The figure shows three views and two pictorial views of one solid part (mm, origin at its lowest corner). Answer the questions. Give positions to 0.01 mm unless a question says otherwise; leave off trailing zeros. Order: outer loops, then holes, each group sorted by start corner. A loop starts at its lowest first (then second) coordinate and runs counter-clockwise, first axis right, second up. Notation, with made-up numbers: (35.5, -11) -> (51.5, -11) arc R19 ccw to (51.5, -6) -> close; hole circle Ø11 at (70.25, -33). An arc over 180 degrees is marked (long way). Use one line per item in the form item = value.
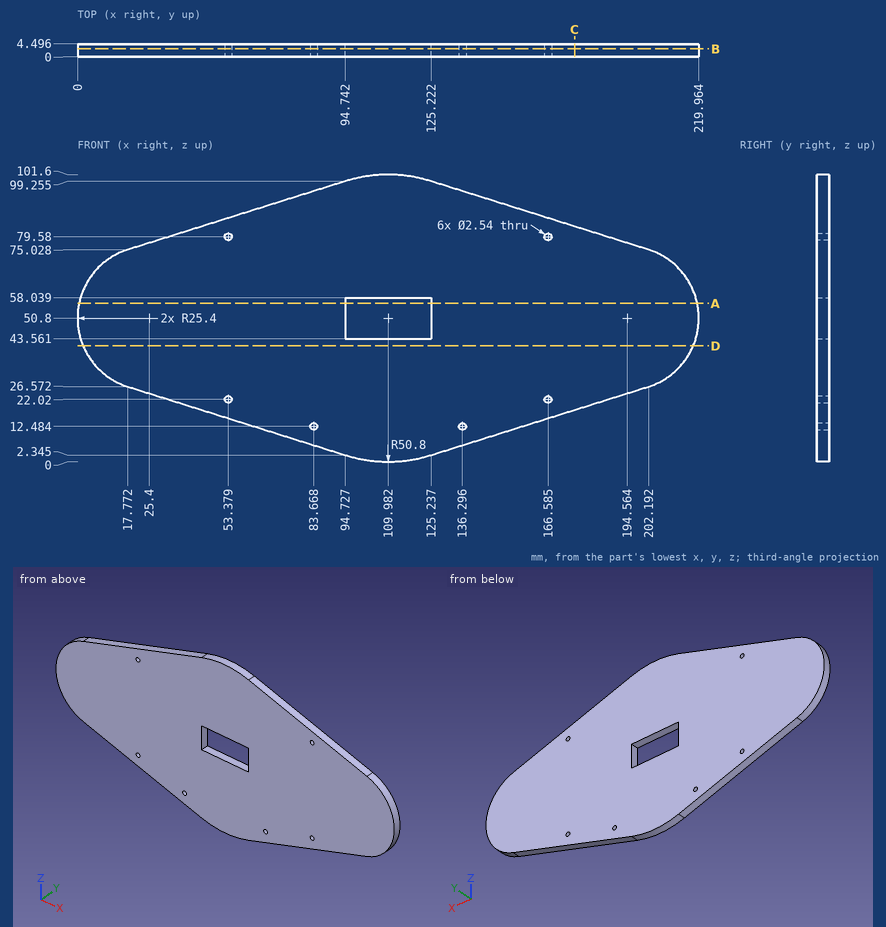
Item 1: The part is cut by section C-C on x = 176. Give the vertices of the cut face in (y, z), and give its area (3 significant figures).
Checks:
outline = (0, 18.33) -> (4.5, 18.33) -> (4.5, 83.27) -> (0, 83.27) -> close
area = 292 mm²
Item 2: Given pin 1 Ø2 at (y, z) = (1, 56.5) entering from -X; pin 2 Ø1.3 at (y, z) = (1.5, 48.5) entering from -X; pin 3 Ø1.5 at (x, y) = (91, 2.5) entering from -Z, each flat-ended and moving along its own axis, determine where each tip first touches the part or whether it passes through.
Checks:
pin_1 = 0.44
pin_2 = 0.05
pin_3 = 3.28
Item 3: Straight lines are drawn through the part: L1, parallel to Z at x = 105, y = 3.5 (1 decimal); L2, parallel to Z at x = 88, y = 4.1; L3, parallel to Z at x = 97.5, y = 4.15. For each, find the intervals that lie inside material, in ascending order. Write a range as from..to.
Checks:
L1 = 0.2..43.6, 58..101.4
L2 = 4.46..97.14
L3 = 1.56..43.56, 58.04..100.04
Item 4: The part is cut by section D-D on z = 41. Give the vertices of the cut face in (x, y).
Checks:
outline = (1.97, 0) -> (218, 0) -> (218, 4.5) -> (1.97, 4.5) -> close
Item 5: The part is cut by section A-A on z = 56. Give the vertices of the cut face in (x, y), and give its area (3 significant figures).
Checks:
outline = (0.54, 0) -> (94.74, 0) -> (94.74, 4.5) -> (0.54, 4.5) -> close; (125.22, 0) -> (219.43, 0) -> (219.43, 4.5) -> (125.22, 4.5) -> close
area = 847 mm²
Item 6: The part is cut by section B-B on y = 2.8. State how many separate pieces and enclosed holes the cut face has, and give its area (3 significant figures).
Checks:
separate_pieces = 1
enclosed_holes = 7
area = 15,000 mm²
